Check sheet for the modelled part. Datum: model origin and axes. Units: mm. A direction names the side the tool comes from. Coordinates: 2 decimals unless noted, no trailing zeros. Loops run counter-clockwise (first coordinate to the right, second up) from the corner with the lowest first, then second, coordinate; pieces in that order, holes last.
```python
from build123d import *

# Parameters (mm, degrees)
F1_DEPTH      = 25
F1_DEPTH_BACK = 25
F2_R          = 17
F3_DEPTH      = 15
F4_R          = 21
F5_DEPTH      = 5
F7_D          = 30
F8_W          = 5
F8_H          = 3
F9_DEPTH      = 5
F10_DEPTH     = 3
F11_D         = 25
F11_DEPTH     = 5
F11_TIP       = 7.5107577378
F12_D         = 8
F13_W         = 3
F13_H         = 20
F14_DEPTH     = 3
F16_D         = 8
F16_DEPTH     = 5
F16_TIP       = 2.4034424761
F18_D         = 8
F18_DEPTH     = 5
F18_TIP       = 2.4034424761
F19_SIZE      = 5
F20_R         = 3


with BuildPart() as f1:
    # F0 (on Front) → F1 (new body, two sides)
    with BuildSketch(Plane.XZ) as f1_sk:
        Polygon((75.3553390593, -35.3553390593), (40, 0), (-40, 0), (-40, -60), (-37, -60), (-37, -3), (38.7573593129, -3), (73.2340187158, -37.4766594029), align=None)
    extrude(amount=F1_DEPTH)
    extrude(f1_sk.sketch, amount=-F1_DEPTH_BACK)

    # F2 (on face) → F3 (join)
    with BuildSketch(Plane.XY):
        Circle(F2_R)
    extrude(amount=F3_DEPTH)

    # F4 (on face) → F5 (join)
    with BuildSketch(Plane(origin=(0, 0, -3), x_dir=(1, 0, 0), z_dir=(0, 0, -1))):
        Circle(F4_R)
    extrude(amount=F5_DEPTH)

    # F7 (through all)
    with Locations(Plane.XY.offset(15)):
        with Locations((0, 0)):
            Hole(F7_D / 2)

    # F8 (on face) → F9 (cut)
    with BuildSketch(Plane(origin=(-40, 0, 0), x_dir=(0, -1, 0), z_dir=(-1, 0, 0))):
        with Locations((27.5, -18.5)):
            Rectangle(F8_W, F8_H)
        with Locations((27.5, -41.5)):
            Rectangle(F8_W, F8_H)
        with Locations((22.5, -18.5)):
            Rectangle(F8_W, F8_H)
        with Locations((22.5, -41.5)):
            Rectangle(F8_W, F8_H)
    extrude(amount=-F9_DEPTH, mode=Mode.SUBTRACT)

    # F8 (on face) → F10 (join)
    with BuildSketch(Plane(origin=(-40, 0, 0), x_dir=(0, -1, 0), z_dir=(-1, 0, 0))):
        with BuildLine():
            Line((-25, -60), (-25, -35))
            ThreePointArc((-25, -35), (-26.4644660941, -38.5355339059), (-30, -40))
            ThreePointArc((-30, -40), (-40, -50), (-30, -60))
            Line((-30, -60), (-25, -60))
        make_face()
        Polygon((0, -30), (-25, -30), (-25, -35), (-25, -60), (0, -60), align=None)
    extrude(amount=-F10_DEPTH)

    # F11
    with Locations(Plane(origin=(-40, 0, 0), x_dir=(0, -1, 0), z_dir=(-1, 0, 0))):
        with Locations((0, -30)):
            Hole(F11_D / 2, depth=F11_DEPTH)
            with Locations((0, 0, -(F11_DEPTH + F11_TIP / 2))):  # 118° drill point
                Cone(0, F11_D / 2, F11_TIP, mode=Mode.SUBTRACT)

    # F12 (through all)
    with Locations(Plane(origin=(-40, 0, 0), x_dir=(0, -1, 0), z_dir=(-1, 0, 0))):
        with Locations((-30, -50)):
            Hole(F12_D / 2)

    # F13 (on face) → F14 (join)
    with BuildSketch(Plane.XZ.offset(25)):
        with BuildLine():
            Line((-25, -20), (-37, -20))
            Line((-37, -20), (-37, -40))
            Line((-37, -40), (-25, -40))
            ThreePointArc((-25, -40), (-15, -30), (-25, -20))
        make_face()
        with Locations((-38.5, -30)):
            Rectangle(F13_W, F13_H)
    extrude(amount=-F14_DEPTH)

    # F16
    with Locations(Plane.XZ.offset(25)):
        with Locations((-25, -30)):
            Hole(F16_D / 2, depth=F16_DEPTH)
            with Locations((0, 0, -(F16_DEPTH + F16_TIP / 2))):  # 118° drill point
                Cone(0, F16_D / 2, F16_TIP, mode=Mode.SUBTRACT)

    # F18
    with Locations(Plane(origin=(20, 0, 20), x_dir=(0.7071067812, 0, -0.7071067812), z_dir=(0.7071067812, 0, 0.7071067812))):
        with Locations((38.2842712475, -15), (38.2842712475, 15), (68.2842712475, -15), (68.2842712475, 15)):
            Hole(F18_D / 2, depth=F18_DEPTH)
            with Locations((0, 0, -(F18_DEPTH + F18_TIP / 2))):  # 118° drill point
                Cone(0, F18_D / 2, F18_TIP, mode=Mode.SUBTRACT)

    # F19
    f19_edges = [f1.edges().sort_by_distance(p)[0] for p in [
        (74.294679, 25, -36.415999),
        (74.294679, -25, -36.415999),
    ]]
    chamfer(f19_edges, length=F19_SIZE)

    # F20
    f20_edges = [f1.edges().sort_by_distance(p)[0] for p in [
        (-40, 0, 0),
        (38.757359, 0, -3),
    ]]
    fillet(f20_edges, radius=F20_R)


solid = f1.part
```
1) Scan lines: line 1 (Y direction, x = 0, z = 9.25); line 2 (Z direction, x = -37.8, y = 30); line 3 (Y direction, x = 0, z = -1). Record each from-to range of solid material in increasing order.
Answer sheet:
line 1: y = -17 to -15, 15 to 17
line 2: z = -60 to -54, -46 to -40
line 3: y = -25 to -15, 15 to 25
2) Section check B-B on x = 0. Enter the section's corners in (y, z).
Answer sheet:
outline: (-25, -3) - (-21, -3) - (-21, -8) - (-15, -8) - (-15, 15) - (-17, 15) - (-17, 0) - (-25, 0) - close; (15, -8) - (21, -8) - (21, -3) - (25, -3) - (25, 0) - (17, 0) - (17, 15) - (15, 15) - close
3) Section check C-C on y = 31.5. Enter the section's corners in (x, z).
Answer sheet:
outline: (-40, -59.89) - (-37, -59.89) - (-37, -53.71) - (-40, -53.71) - close; (-40, -46.29) - (-37, -46.29) - (-37, -40.11) - (-40, -40.11) - close
4) Set-up check for faces 5 (the cylindrical face through (-15, -24, -30)), 6 (the cylindrical face through (-38.479, -2.71, -42.203)), 7 (the cylindrical face through (9.139, 14.334, 7.395)), 8 (the flat face through (56.2, -0.35, -20.44)), 9 (the cylindrical face through (20.03, -6.31, -5.46)): record each of +Z, -Z, +X, -X, +Y, -Y from which the full face is reachable in a straight line by a thin tool's end or side.
Answer sheet:
face 5: +Y, -Y
face 6: -X
face 7: +Z
face 8: -Z, +Y, -Y
face 9: -Z
5) Depth check by flat-ended pin: pin 1 (0.9 mm diameter, centred on x = -38, z = -19, fed in from -Y); pin 2 (2 mm diameter, centred on y = 27.5, z = -20, fed in from +X); pin 3 (10 mm diameter, centred on x = 34.5, y = 2, fed in from +Z); pin 4 (13 mm diameter, centred on x = -25, z = -30, fed in from +Y). Enter the tip coordinate at first touch or a pass-through.
Answer sheet:
pin 1: stops at y = -20
pin 2: passes through
pin 3: stops at z = 0
pin 4: stops at y = -22
6) Section check D-D on x = 23.5. Enter the section's corners in (y, z), plus the area to 3 significant figures.
Answer sheet:
outline: (-25, -3) - (25, -3) - (25, 0) - (-25, 0) - close
area: 150 mm2
7) Mould release check, pull along Z, two halves, no side actions. Record for faces 1 (the flat face through (-39, -23, -17)), 2 (the cylindrical face through (-38.5, 26.8, -52.4)), 3 (the flat face through (72.54, 22.46, -34.69)), 4 (the flat face through (-39, -25, -51)): +Z half, -Z half, draft (parallel to the pull), parting line (faces both ways), or undercut.
Answer sheet:
face 1: undercut
face 2: undercut
face 3: -Z half
face 4: draft
8) Section check A-A on y = 0. Enter the section's corners in (x, z).
Answer sheet:
outline: (-40, -60) - (-37, -60) - (-37, -42.5) - (-40, -42.5) - close; (-40, -17.5) - (-37, -17.5) - (-37, -3) - (-21, -3) - (-21, -8) - (-15, -8) - (-15, 15) - (-17, 15) - (-17, 0) - (-37, 0) arc R3 ccw to (-40, -3) - close; (15, -8) - (21, -8) - (21, -3) - (37.51, -3) arc R3 cw to (39.64, -3.88) - (73.23, -37.48) - (75.36, -35.36) - (40, 0) - (17, 0) - (17, 15) - (15, 15) - close
